The listing builds one solid part. Answer for the finished solid, in the listing's coordinates (mm). Face numbers are marked on the shaded views. A direction names the side the tool comes from. Round coordinates to 2 decimals unless told otherwise and drop trailing zeros. Write each loop counter-clockwise with the first axis right and the second up, starting at its lowest first coordinate (ties: lowest second). Pieces come first, ordered by that corner, then holes. Notation, with made-up numbers: M 77.5,-25.75 L 105.5,-25.75 A20 ccw 105.5,5.25 Z; hole C 40,63 d6. An arc over 180 degrees is marked long. One line per item, written item: value. Start each with the question number.
(1) For the marked faces 5, 6 and 7, determine the directions among +Z, -Z, +X, -X, +Y, -Y from which every point of the face is accessible in a straight line to the end or side of a thin tool.
(2) Given P1, Ø6, axis at y = 6, z = 10.5, coming from the -X side; P2, Ø12, axis at y = 2.5, z = -6.5, coming from the -X side; P3, Ø4.5, axis at x = -5, z = 3.5, coming from the +Y side; P4, Ø4, axis at x = -24.3, y = -16.98, coming from the -Z side, each flat-ended and moving along its own axis, determine where each tip first touches the part or whether it passes through.
(3) Section D-D (x = 15.5) is taken. Determine the outline of the cut face in (y, z), plus the area to 3 significant figures.
(4) For a pull along Z with two mould halves and no side action, classify the marked faces 1, 2, 3 and 4 as released by +Z, released by -Z, zero draft, split by the parting line, or undercut.
(5) Section A-A (y = -20) is taken. Determine the outline of the cut face in (x, z).
(6) Section C-C (x = -50.5) is taken. Determine the outline of the cut face in (y, z), plus the area to 3 significant figures.
(7) Consider probe 1 along Z at (x, y) = (-15, -19); probe 2 along Z at (x, y) = (22, 24.5); probe 3 along Y at (x, z) = (-34, -3.5). Determine where each line is inside the solid, lowest interval first.
(8) Section B-B (z = 2.5) is taken. Determine the outline of the cut face in (x, y).
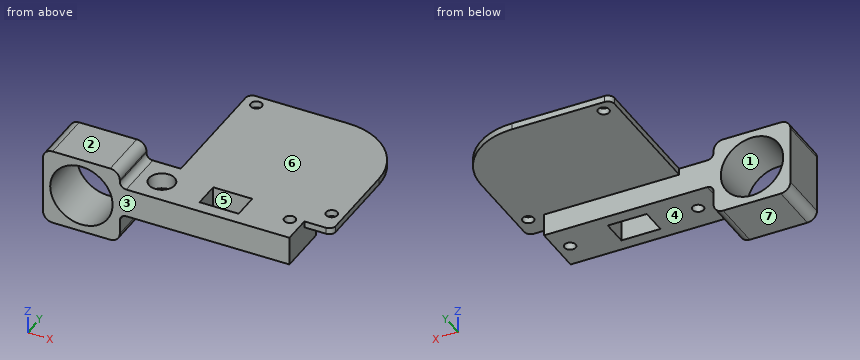
```python
from build123d import *

# Parameters (mm, degrees)
F0_R            = 1.75
F0_W            = 12.2
F0_H            = 8.2
F1_DEPTH        = 9
F2_R            = 9.75
F3_DEPTH        = 16
F4_R            = 3
F6_R            = 2
F7_R            = 1.75
F8_DEPTH        = 2
F9_DEPTH        = 2
F10_R           = 2
F11_R           = 20
F13_D           = 3.5
F13_CBORE_D     = 8
F13_CBORE_DEPTH = 5


with BuildPart() as f1:
    # F0 (on Top) → F1 (new body)
    with BuildSketch(Plane.XY):
        Polygon((19.6991001874, -8.9786109865), (-33.3008998126, -8.9786109865), (-33.3008998126, -24.9786109865), (-24.3008998126, -24.9786109865), (19.6991001874, -24.9786109865), align=None)
        with Locations((-24.3008998126, -16.9786109865)):
            Circle(F0_R, mode=Mode.SUBTRACT)
        with Locations((-4.3008998126, -16.9786109865)):
            Rectangle(F0_W, F0_H, mode=Mode.SUBTRACT)
        with Locations((15.6991001874, -16.9786109865)):
            Circle(F0_R, mode=Mode.SUBTRACT)
    extrude(amount=F1_DEPTH)


with BuildPart() as f3:
    # F2 (on face) → F3 (new body)
    with BuildSketch(Plane(origin=(0, -8.9786109865, 0), x_dir=(-1, 0, 0), z_dir=(0, 1, 0))):
        Polygon((33.3008998126, 9), (33.3008998126, 0), (33.3008998126, -9.5), (57.3008998126, -9.5), (57.3008998126, 14.5), (33.3008998126, 14.5), align=None)
        with Locations((45.3008998126, 2.5)):
            Circle(F2_R, mode=Mode.SUBTRACT)
    extrude(amount=-F3_DEPTH)

    # F4
    f4_edges = [f3.edges().sort_by_distance(p)[0] for p in [
        (-33.3009, -16.978611, 14.5),
        (-57.3009, -16.978611, 14.5),
        (-57.3009, -16.978611, -9.5),
        (-33.3009, -16.978611, -9.5),
    ]]
    fillet(f4_edges, radius=F4_R)


with BuildPart() as f1_1:
    add(f1.part)

    # F5: union F3
    add(f3.part)

    # F6
    f6_edges = [f1_1.edges().sort_by_distance(p)[0] for p in [
        (-33.3009, -16.978611, 0),
        (-33.3009, -16.978611, 9),
    ]]
    fillet(f6_edges, radius=F6_R)

    # F7 (on face) → F8 (join)
    with BuildSketch(Plane.XY.offset(9)):
        Polygon((19.6991001874, -8.9786109865), (19.6991001874, -15.9786109865), (28.4491001874, -15.9786109865), (28.4491001874, 32.0213890135), (-22.5508998126, 32.0213890135), (-22.5508998126, -8.9786109865), align=None)
        with Locations((24.6991001874, -9.1451848542)):
            Circle(F7_R, mode=Mode.SUBTRACT)
        with Locations((-18.3008998126, 28.2713890135)):
            Circle(F7_R, mode=Mode.SUBTRACT)
        with Locations((-18.3008998126, 28.2713890135)):
            Circle(F7_R)
        with Locations((24.6991001874, -9.1451848542)):
            Circle(F7_R)
    extrude(amount=-F8_DEPTH)

    # F7 (on face) → F9 (cut, through all)
    with BuildSketch(Plane.XY.offset(9)):
        with Locations((-18.3008998126, 28.2713890135)):
            Circle(F7_R)
        with Locations((24.6991001874, -9.1451848542)):
            Circle(F7_R)
    extrude(amount=-F9_DEPTH, mode=Mode.SUBTRACT)

    # F10
    f10_edges = [f1_1.edges().sort_by_distance(p)[0] for p in [
        (-22.5509, 32.021389, 8),
        (28.4491, -15.978611, 8),
    ]]
    fillet(f10_edges, radius=F10_R)

    # F11
    f11_edges = [f1_1.edges().sort_by_distance(p)[0] for p in [
        (28.4491, 32.021389, 8),
    ]]
    fillet(f11_edges, radius=F11_R)

    # F13 (through all)
    with Locations(Plane.XY.offset(9)):
        with Locations((-24.3008998126, -16.9786109865)):
            CounterBoreHole(F13_D / 2, F13_CBORE_D / 2, F13_CBORE_DEPTH)


solid = f1_1.part
```
Recorded:
1. face 5: +Z, -Z
1. face 6: +Z, +X, +Y, -Y
1. face 7: -Z, +X, -X, +Y, -Y
2. P1: stops at x = -22.55
2. P2: passes through
2. P3: stops at y = -8.98
2. P4: stops at z = 0
3. outline: M -24.98,0 L -18.72,0 L -18.72,9 L -24.98,9 Z; M -15.24,0 L -8.98,0 L -8.98,7 L 30.74,7 L 30.74,9 L -15.24,9 Z
3. area: 192 mm2
4. face 1: undercut
4. face 2: released by +Z
4. face 3: zero draft
4. face 4: released by -Z
5. outline: M -57.3,-6.5 A3 ccw -54.3,-9.5 L -36.3,-9.5 A3 ccw -33.3,-6.5 L -33.3,-2 A2 cw -31.3,0 L -10.4,0 L -10.4,9 L -21.68,9 L -21.68,4 L -26.92,4 L -26.92,9 L -31.3,9 A2 cw -33.3,11 L -33.3,11.5 A3 ccw -36.3,14.5 L -54.3,14.5 A3 ccw -57.3,11.5 Z; M 1.8,0 L 19.7,0 L 19.7,9 L 1.8,9 Z; hole C -45.3,2.5 d19.5
6. outline: M -24.98,-9.5 L -8.98,-9.5 L -8.98,-5.75 L -24.98,-5.75 Z; M -24.98,10.75 L -8.98,10.75 L -8.98,14.5 L -24.98,14.5 Z
6. area: 120 mm2
7. probe 1: z = 0 to 9
7. probe 2: z = 7 to 9
7. probe 3: y = -24.98 to -8.98
8. outline: M -57.3,-24.98 L -55.05,-24.98 L -55.05,-8.98 L -57.3,-8.98 Z; M -35.55,-24.98 L 19.7,-24.98 L 19.7,-8.98 L -35.55,-8.98 Z; hole C -24.3,-16.98 d3.5; hole M -10.4,-21.08 L 1.8,-21.08 L 1.8,-12.88 L -10.4,-12.88 Z; hole C 15.7,-16.98 d3.5
